The figure shows three views and two pictorial views of one solid part (mm, origin at its lowest corner). Answer the questions. A direction names the side the tool comes from. Round coordinates to 2 decimals unless told otherwise and drop trailing zeros. Order: outer loops, then holes, each group sorted by start corner. A loop starts at its lowest first (then second) coordinate and runs counter-clockwise, first axis right, second up. Notation, with made-up numbers: (-28, 53.25) - (17, 53.25) arc R29 ccw to (17, 78.25) - close; hole circle Ø1 at (-15.5, 55). An arc over 180 degrees is marked (long way). Answer as a JSON object with one key per item and string values. Group by question number.
Q1. The mould has two halves that part along Z. Classify the marked faces 1, 2, 3 and 4: pulls with the +Z half, pulls with the -Z half, needs draft (parallel to the pull), parting line crosses it, or undercut.
Q2. A tool of negligible diameter and unlimited length cuts with its end or side. For the marked faces 5 and 6, from which of +Z, -Z, +X, -X, +Y, -Y can it reach the whole face along a straight path? Write none if from no direction.
Q3. A cutting plane is placed at B-B on z = 12.5. Determine the outline of the cut face in (x, y).
Q4. A cutting plane is placed at C-C on y = 6.75. Determine the outline of the cut face in (x, z).
Q5. Consider line 1 (Z direction, x = 10, y = 17.5); line 2 (X direction, y = 16.25, z = 12.5); line 3 (Y direction, x = 19, z = 12). Determine where each line is inside the solid, lowest interval first.
Q6. Given pin 1 Ø5 at (y, z) = (6, 5) entering from -X; pin 2 Ø1 at (x, z) = (18, 14) entering from -Y, each flat-ended and moving along its own axis, determine where each tip first touches the part or whether it passes through.
Q7. A cutting plane is placed at A-A on x = 10. Determine the outline of the cut face in (y, z).
Q8. A cutting plane is placed at D-D on z = 3.5. Determine the outline of the cut face in (x, y), and give its area (3 significant figures).
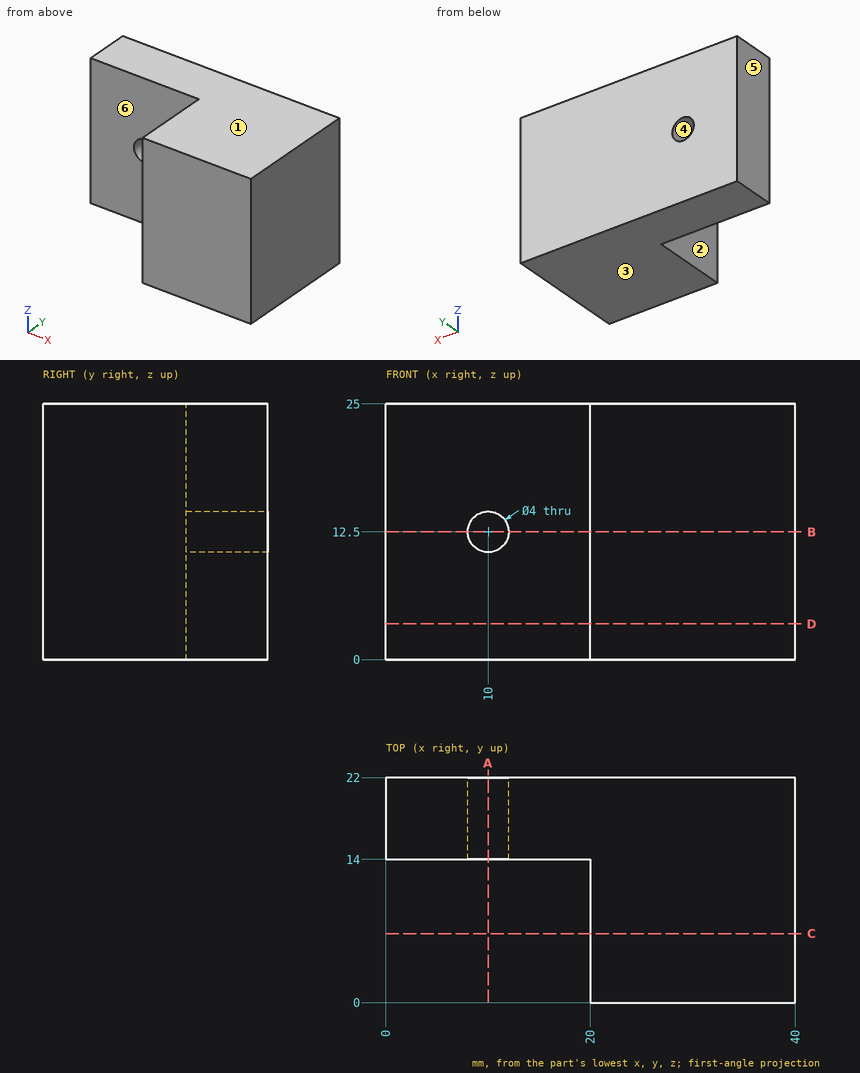
Result set:
{
 "1": {"face 1": "pulls with the +Z half", "face 2": "needs draft", "face 3": "pulls with the -Z half", "face 4": "undercut"},
 "2": {"face 5": "+Z, -Z, -X, +Y, -Y", "face 6": "+Z, -Z, -X, -Y"},
 "3": {"outline": "(0, 14) - (8, 14) - (8, 22) - (0, 22) - close; (12, 14) - (20, 14) - (20, 0) - (40, 0) - (40, 22) - (12, 22) - close"},
 "4": {"outline": "(20, 0) - (40, 0) - (40, 25) - (20, 25) - close"},
 "5": {"line 1": "z = 0 to 10.5, 14.5 to 25", "line 2": "x = 0 to 8, 12 to 40", "line 3": "y = 14 to 22"},
 "6": {"pin 1": "stops at x = 20", "pin 2": "stops at y = 14"},
 "7": {"outline": "(14, 0) - (22, 0) - (22, 10.5) - (14, 10.5) - close; (14, 14.5) - (22, 14.5) - (22, 25) - (14, 25) - close"},
 "8": {"outline": "(0, 14) - (20, 14) - (20, 0) - (40, 0) - (40, 22) - (0, 22) - close", "area": "600 mm²"}
}
